Could you check a few things on this model? Use its own coordinates, in mm. Coordinates: 2 decimals unless noted, no trailing zeros. Order: outer loops, then holes, each group sorted by start corner. A loop starts at its lowest first (then second) coordinate and runs counter-clockwise, first axis right, second up. Notation, with made-up numbers: (-19, 17.25) - (21, 17.25) arc R29 cw to (21, 52.25) - close; hole circle Ø10 at (-33, 11). An arc over 180 degrees is marked (long way). Answer as a JSON object with one key per item and string values. Group by question number.
(1) Imagine slicing it at A-A, the plane y = 4.25. Write out the boundary of the cut face in (x, z) (3 decimals).
(2) Imagine slicing it at D-D, the plane z = -61.5. Write out the boundary of the cut face in (x, y), and give its area (3 significant figures).
(3) Please list where these lines run through material, in increasing order: probe 1 along X at (y, z) = (-1.9, -15.25) (3 decimals); probe 2 along X at (y, z) = (-1, 25.5) (3 decimals); probe 3 along X at (y, z) = (5, -40) (3 decimals).
(4) Will these pins go through, and if not, where does the flat tip stop? P1, Ø1.8, axis at y = 4, z = -3.5, coming from the +X side (3 decimals); P2, Ø2.5, axis at x = 18.5, y = 2.5, coming from the -Z side; P3, Ø6.5, axis at x = 55.96, z = -67.27, coming from the +Y side; P4, Ø2.5, axis at x = -15.25, z = 15.25, coming from the +Y side.
(5) Imagine slicing it at C-C, the plane x = -50. Write out the boundary of the cut face in (y, z).
(6) Imagine slicing it at B-B, the plane z = -38.5. Write out the boundary of the cut face in (x, y) (3 decimals).
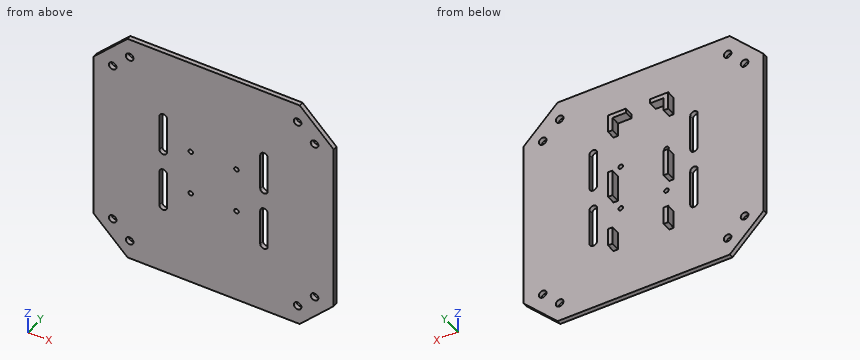
from build123d import *

# Parameters (mm, degrees)
SKETCH1_W                                  = 160
SKETCH1_H                                  = 160
BOSS_EXTRUDE1_DEPTH                        = 3
CUT_EXTRUDE2_REACH                         = 115.177
CUT_EXTRUDE1_REACH                         = 115.177
SKETCH2_R                                  = 2.55
MIRROR2_AT_THE_SECOND_PLANE_COPY_1_REACH   = 115.177
MIRROR2_AT_THE_SECOND_PLANE_COPY_2_REACH   = 115.177
MIRROR2_AT_THE_SECOND_PLANE_COPY_2_SKETC_R = 2.55
CUT_EXTRUDE3_REACH                         = 115.177
SKETCH11_R                                 = 1.525
SKETCH12_W                                 = 3
SKETCH12_H                                 = 12
SKETCH12_H_2                               = 18
BOSS_EXTRUDE2_DEPTH                        = 6
CUT_EXTRUDE4_REACH                         = 115.296
MIRROR4_AT_THE_SECOND_PLANE_COPY_1_REACH   = 115.296


with BuildPart() as part:
    # Sketch1 → Boss-Extrude1 (new body)
    with BuildSketch(Plane(origin=(0, 0, 0), x_dir=(1, 0, 0), z_dir=(0, 1, 0))):
        Rectangle(SKETCH1_W, SKETCH1_H)
    extrude(amount=-BOSS_EXTRUDE1_DEPTH)

    # Sketch6 → Cut-Extrude2 (cut, up to next)
    with BuildSketch(Plane(origin=(0, 0, 0), x_dir=(1, 0, 0), z_dir=(0, 1, 0)), mode=Mode.PRIVATE) as cut_extrude2_sk1:
        Polygon((-80, -57.372583002), (-57.372583002, -80), (-80, -80), align=None)
    cut_extrude2_tool1 = extrude(cut_extrude2_sk1.sketch, amount=-CUT_EXTRUDE2_REACH, mode=Mode.PRIVATE) & part.part
    cut_extrude2 = cut_extrude2_tool1.solids().sort_by_distance((-72.457528, 0, 72.457528))[0]
    add(cut_extrude2, mode=Mode.SUBTRACT)

    # Sketch2 → Cut-Extrude1 (cut, up to next)
    with BuildSketch(Plane(origin=(0, 0, 0), x_dir=(1, 0, 0), z_dir=(0, 1, 0)), mode=Mode.PRIVATE) as cut_extrude1_sk1:
        with Locations(Location((-67.272077939, -55.95836944, 0), (0, 0, 270))):
            Circle(SKETCH2_R)
    cut_extrude1_tool1 = extrude(cut_extrude1_sk1.sketch, amount=-CUT_EXTRUDE1_REACH, mode=Mode.PRIVATE) & part.part
    # Sketch2 → Cut-Extrude1 (cut, up to next)
    with BuildSketch(Plane(origin=(0, 0, 0), x_dir=(1, 0, 0), z_dir=(0, 1, 0)), mode=Mode.PRIVATE) as cut_extrude1_sk2:
        with Locations(Location((-55.95836944, -67.272077939, 0), (0, 0, 270))):
            Circle(SKETCH2_R)
    cut_extrude1_tool2 = extrude(cut_extrude1_sk2.sketch, amount=-CUT_EXTRUDE1_REACH, mode=Mode.PRIVATE) & part.part
    cut_extrude1_1 = cut_extrude1_tool1.solids().sort_by_distance((-67.272078, 0, 55.958369))[0]
    add(cut_extrude1_1, mode=Mode.SUBTRACT)
    cut_extrude1_2 = cut_extrude1_tool2.solids().sort_by_distance((-55.958369, 0, 67.272078))[0]
    add(cut_extrude1_2, mode=Mode.SUBTRACT)
    cut_extrude1 = cut_extrude1_1 + cut_extrude1_2  # Cut-Extrude1 as one shape, for the pattern or mirror that repeats it

    # Mirror2: Cut-Extrude2, Cut-Extrude1 across plane
    add(cut_extrude2.mirror(Plane(origin=(0, 0, 0), x_dir=(0, 0, 1), z_dir=(1, 0, 0))), mode=Mode.SUBTRACT)
    add(cut_extrude1.mirror(Plane(origin=(0, 0, 0), x_dir=(0, 0, 1), z_dir=(1, 0, 0))), mode=Mode.SUBTRACT)

    # Mirror2 at the second plane: Cut-Extrude2, Cut-Extrude1 across plane
    add(cut_extrude2.mirror(Plane.XY), mode=Mode.SUBTRACT)
    add(cut_extrude1.mirror(Plane.XY), mode=Mode.SUBTRACT)

    # Mirror2 at the second plane copy 1 sketc → Mirror2 at the second plane copy 1 (cut, up to next)
    with BuildSketch(Plane(origin=(0, 0, 0), x_dir=(-1, 0, 0), z_dir=(0, 1, 0)), mode=Mode.PRIVATE) as mirror2_at_the_second_plane_copy_1_sk1:
        Polygon((-80, -57.372583002), (-57.372583002, -80), (-80, -80), align=None)
    mirror2_at_the_second_plane_copy_1_tool1 = extrude(mirror2_at_the_second_plane_copy_1_sk1.sketch, amount=-MIRROR2_AT_THE_SECOND_PLANE_COPY_1_REACH, mode=Mode.PRIVATE) & part.part
    add(mirror2_at_the_second_plane_copy_1_tool1.solids().sort_by_distance((72.457528, 0, -72.457528))[0], mode=Mode.SUBTRACT)

    # Mirror2 at the second plane copy 2 sketc → Mirror2 at the second plane copy 2 (cut, up to next)
    with BuildSketch(Plane(origin=(0, 0, 0), x_dir=(-1, 0, 0), z_dir=(0, 1, 0)), mode=Mode.PRIVATE) as mirror2_at_the_second_plane_copy_2_sk1:
        with Locations(Location((-67.272077939, -55.95836944, 0), (0, 0, 270))):
            Circle(MIRROR2_AT_THE_SECOND_PLANE_COPY_2_SKETC_R)
    mirror2_at_the_second_plane_copy_2_tool1 = extrude(mirror2_at_the_second_plane_copy_2_sk1.sketch, amount=-MIRROR2_AT_THE_SECOND_PLANE_COPY_2_REACH, mode=Mode.PRIVATE) & part.part
    # Mirror2 at the second plane copy 2 sketc → Mirror2 at the second plane copy 2 (cut, up to next)
    with BuildSketch(Plane(origin=(0, 0, 0), x_dir=(-1, 0, 0), z_dir=(0, 1, 0)), mode=Mode.PRIVATE) as mirror2_at_the_second_plane_copy_2_sk2:
        with Locations(Location((-55.95836944, -67.272077939, 0), (0, 0, 270))):
            Circle(MIRROR2_AT_THE_SECOND_PLANE_COPY_2_SKETC_R)
    mirror2_at_the_second_plane_copy_2_tool2 = extrude(mirror2_at_the_second_plane_copy_2_sk2.sketch, amount=-MIRROR2_AT_THE_SECOND_PLANE_COPY_2_REACH, mode=Mode.PRIVATE) & part.part
    add(mirror2_at_the_second_plane_copy_2_tool1.solids().sort_by_distance((67.272078, 0, -55.958369))[0], mode=Mode.SUBTRACT)
    add(mirror2_at_the_second_plane_copy_2_tool2.solids().sort_by_distance((55.958369, 0, -67.272078))[0], mode=Mode.SUBTRACT)

    # Sketch11 → Cut-Extrude3 (cut, up to next)
    with BuildSketch(Plane(origin=(0, 0, 0), x_dir=(1, 0, 0), z_dir=(0, 1, 0)), mode=Mode.PRIVATE) as cut_extrude3_sk1:
        with Locations(Location((-15.25, 15.25, 0), (0, 0, 270))):
            Circle(SKETCH11_R)
    cut_extrude3_tool1 = extrude(cut_extrude3_sk1.sketch, amount=-CUT_EXTRUDE3_REACH, mode=Mode.PRIVATE) & part.part
    # Sketch11 → Cut-Extrude3 (cut, up to next)
    with BuildSketch(Plane(origin=(0, 0, 0), x_dir=(1, 0, 0), z_dir=(0, 1, 0)), mode=Mode.PRIVATE) as cut_extrude3_sk2:
        with Locations(Location((15.25, 15.25, 0), (0, 0, 270))):
            Circle(SKETCH11_R)
    cut_extrude3_tool2 = extrude(cut_extrude3_sk2.sketch, amount=-CUT_EXTRUDE3_REACH, mode=Mode.PRIVATE) & part.part
    # Sketch11 → Cut-Extrude3 (cut, up to next)
    with BuildSketch(Plane(origin=(0, 0, 0), x_dir=(1, 0, 0), z_dir=(0, 1, 0)), mode=Mode.PRIVATE) as cut_extrude3_sk3:
        with Locations(Location((15.25, -15.25, 0), (0, 0, 270))):
            Circle(SKETCH11_R)
    cut_extrude3_tool3 = extrude(cut_extrude3_sk3.sketch, amount=-CUT_EXTRUDE3_REACH, mode=Mode.PRIVATE) & part.part
    # Sketch11 → Cut-Extrude3 (cut, up to next)
    with BuildSketch(Plane(origin=(0, 0, 0), x_dir=(1, 0, 0), z_dir=(0, 1, 0)), mode=Mode.PRIVATE) as cut_extrude3_sk4:
        with Locations(Location((-15.25, -15.25, 0), (0, 0, 270))):
            Circle(SKETCH11_R)
    cut_extrude3_tool4 = extrude(cut_extrude3_sk4.sketch, amount=-CUT_EXTRUDE3_REACH, mode=Mode.PRIVATE) & part.part
    add(cut_extrude3_tool1.solids().sort_by_distance((-15.25, 0, -15.25))[0], mode=Mode.SUBTRACT)
    add(cut_extrude3_tool2.solids().sort_by_distance((15.25, 0, -15.25))[0], mode=Mode.SUBTRACT)
    add(cut_extrude3_tool3.solids().sort_by_distance((15.25, 0, 15.25))[0], mode=Mode.SUBTRACT)
    add(cut_extrude3_tool4.solids().sort_by_distance((-15.25, 0, 15.25))[0], mode=Mode.SUBTRACT)

    # Sketch12 → Boss-Extrude2 (add)
    with BuildSketch(Plane(origin=(0, 0, 0), x_dir=(1, 0, 0), z_dir=(0, 1, 0))):
        Polygon((-17.075, -47.55), (-8.075, -47.55), (-8.075, -50.55), (-20.075, -50.55), (-20.075, -38.55), (-17.075, -38.55), align=None)
        with Locations((-18.575, 38.55)):
            Rectangle(SKETCH12_W, SKETCH12_H)
        with Locations((-18.575, 0)):
            Rectangle(SKETCH12_W, SKETCH12_H_2)
    boss_extrude2 = extrude(amount=BOSS_EXTRUDE2_DEPTH)

    # Mirror3: Boss-Extrude2 across plane
    add(boss_extrude2.mirror(Plane(origin=(0, 0, 0), x_dir=(0, 0, 1), z_dir=(1, 0, 0))))

    # Sketch13 → Cut-Extrude4 (cut, up to next)
    with BuildSketch(Plane(origin=(0, 0, 0), x_dir=(1, 0, 0), z_dir=(0, 1, 0)), mode=Mode.PRIVATE) as cut_extrude4_sk1:
        with BuildLine():
            Line((-31.075, 32.55), (-31.075, 8))
            ThreePointArc((-31.075, 8), (-33.575, 5.5), (-36.075, 8))
            Line((-36.075, 8), (-36.075, 32.55))
            ThreePointArc((-36.075, 32.55), (-33.575, 35.05), (-31.075, 32.55))
        make_face()
    cut_extrude4_tool1 = extrude(cut_extrude4_sk1.sketch, amount=-CUT_EXTRUDE4_REACH, mode=Mode.PRIVATE) & part.part
    cut_extrude4 = cut_extrude4_tool1.solids().sort_by_distance((-33.575, 0, -20.275))[0]
    add(cut_extrude4, mode=Mode.SUBTRACT)

    # Mirror4: Cut-Extrude4 across plane
    add(cut_extrude4.mirror(Plane(origin=(0, 0, 0), x_dir=(0, 0, 1), z_dir=(1, 0, 0))), mode=Mode.SUBTRACT)

    # Mirror4 at the second plane: Cut-Extrude4 across plane
    add(cut_extrude4.mirror(Plane.XY), mode=Mode.SUBTRACT)

    # Mirror4 at the second plane copy 1 sketc → Mirror4 at the second plane copy 1 (cut, up to next)
    with BuildSketch(Plane(origin=(0, 0, 0), x_dir=(-1, 0, 0), z_dir=(0, 1, 0)), mode=Mode.PRIVATE) as mirror4_at_the_second_plane_copy_1_sk1:
        with BuildLine():
            Line((-31.075, 32.55), (-31.075, 8))
            ThreePointArc((-31.075, 8), (-33.575, 5.5), (-36.075, 8))
            Line((-36.075, 8), (-36.075, 32.55))
            ThreePointArc((-36.075, 32.55), (-33.575, 35.05), (-31.075, 32.55))
        make_face()
    mirror4_at_the_second_plane_copy_1_tool1 = extrude(mirror4_at_the_second_plane_copy_1_sk1.sketch, amount=-MIRROR4_AT_THE_SECOND_PLANE_COPY_1_REACH, mode=Mode.PRIVATE) & part.part
    add(mirror4_at_the_second_plane_copy_1_tool1.solids().sort_by_distance((33.575, 0, 20.275))[0], mode=Mode.SUBTRACT)


solid = part.part
Result set:
{
 "1": {"outline": "(-20.075, -44.55) - (-17.075, -44.55) - (-17.075, -32.55) - (-20.075, -32.55) - close; (-20.075, -9) - (-17.075, -9) - (-17.075, 9) - (-20.075, 9) - close; (-20.075, 38.55) - (-17.075, 38.55) - (-17.075, 47.55) - (-8.075, 47.55) - (-8.075, 50.55) - (-20.075, 50.55) - close; (8.075, 47.55) - (17.075, 47.55) - (17.075, 38.55) - (20.075, 38.55) - (20.075, 50.55) - (8.075, 50.55) - close; (17.075, -44.55) - (20.075, -44.55) - (20.075, -32.55) - (17.075, -32.55) - close; (17.075, -9) - (20.075, -9) - (20.075, 9) - (17.075, 9) - close"},
 "2": {"outline": "(-75.87, -3) - (75.87, -3) - (75.87, 0) - (-75.87, 0) - close", "area": "455 mm^2"},
 "3": {"probe 1": "x = -80 to -36.075, -31.075 to -16.775, -13.725 to 13.725, 16.775 to 31.075, 36.075 to 80", "probe 2": "x = -80 to -36.075, -31.075 to 31.075, 36.075 to 80", "probe 3": "x = -20.075 to -17.075, 17.075 to 20.075"},
 "4": {"P1": "stops at x = 20.075", "P2": "stops at z = -44.55", "P3": "stops at y = 0", "P4": "passes through"},
 "5": {"outline": "(-3, -80) - (0, -80) - (0, 80) - (-3, 80) - close"},
 "6": {"outline": "(-80, -3) - (80, -3) - (80, 0) - (20.075, 0) - (20.075, 6) - (17.075, 6) - (17.075, 0) - (-17.075, 0) - (-17.075, 6) - (-20.075, 6) - (-20.075, 0) - (-80, 0) - close"}
}
